Design review of the part built by this model. Coordinates are the model's own, in mm. Face numbers are marked on the shaded views. A direction names the side the tool comes from. Coordinates: 2 decimals unless noted, no trailing zeros. Write each loop counter-clockwise with the first axis right and the second up, starting at its lowest first coordinate (ties: lowest second). Pieces come first, ordered by that corner, then holes.
Q1. For pin 1 Ø2 at (y, z) = (-8.5, -12) entering from -X; pin 2 Ø1 at (x, z) = (-1.5, 6.5) entering from -Y; pin 3 Ø1 at (y, z) = (5, 30) entering from +X, all flat-tipped, find the tip position at first contact; note any pin that passes through.
Q2. Take a section at D-D, the plane x = 6. Write out the cut boundary in (y, z), plus the area to 3 significant figures.
Q3. Take a section at C-C, the plane y = 2.5. Write out the cut boundary in (x, z), plus the area to 3 significant figures.
Q4. For L1, parallel to Y at x = -1.5, z = 33; L2, parallel to Z at x = -4.75, y = 9; L3, parallel to Y at x = -1.9, z = 30.5, list the stretches that pass through material, from the lowest coordinate up.
Q5. For the marked faces 1, 2 and 3, list the 3-axis set-ups (+Z, -Z, +X, -X, +Y, -Y) from which the entire face can be reached by the end or side of a thin tool; tool diameter is ignored.
Q6. Take a section at A-A, the plane z = 61.5. Write out the cut boundary in (x, y).
Q7. Take a section at B-B, the plane z = -12. Write out the cut boundary in (x, y).
from build123d import *

# Parameters (mm, degrees)
SKETCH2_W                                    = 26
SKETCH2_H                                    = 43.2
BOSS_EXTRUDE1_DEPTH                          = 10.1
SKETCH3_R                                    = 1.75
BOSS_EXTRUDE2_DEPTH                          = 7
BOSS_EXTRUDE3_DEPTH                          = 26
BOSS_EXTRUDE4_DEPTH                          = 7
CHAMFER1_SIZE                                = 4.24
CBORE_FOR_M5_HEX_HEAD_CAP_SCREW1_D           = 3.9
CBORE_FOR_M5_HEX_HEAD_CAP_SCREW1_CBORE_D     = 6
CBORE_FOR_M5_HEX_HEAD_CAP_SCREW1_CBORE_DEPTH = 4


with BuildPart() as part:
    # Sketch2 → Boss-Extrude1 (new body)
    with BuildSketch(Plane(origin=(0, 0, 0), x_dir=(0, 0, -1), z_dir=(1, 0, 0))):
        Rectangle(SKETCH2_W, SKETCH2_H)
    extrude(amount=BOSS_EXTRUDE1_DEPTH)

    # Sketch3 → Boss-Extrude2 (add)
    with BuildSketch(Plane.ZY):
        Polygon((-17.5, 15), (17.5, 15), (62.5, 15), (62.5, -15), (17.5, -15), (-17.5, -15), align=None)
        with Locations(Location((12, 9, 0), (0, 0, 304.849904579))):
            Circle(SKETCH3_R, mode=Mode.SUBTRACT)
        with Locations(Location((12, -9, 0), (0, 0, 55.150095421))):
            Circle(SKETCH3_R, mode=Mode.SUBTRACT)
        with Locations(Location((-12, -9, 0), (0, 0, 124.849904579))):
            Circle(SKETCH3_R, mode=Mode.SUBTRACT)
        with Locations(Location((-12, 9, 0), (0, 0, 124.849904579))):
            Circle(SKETCH3_R, mode=Mode.SUBTRACT)
        with Locations(Location((57, -9, 0), (0, 0, 180))):
            Circle(SKETCH3_R, mode=Mode.SUBTRACT)
        with Locations(Location((57, 9, 0), (0, 0, 180))):
            Circle(SKETCH3_R, mode=Mode.SUBTRACT)
        with Locations(Location((33, -9, 0), (0, 0, 180))):
            Circle(SKETCH3_R, mode=Mode.SUBTRACT)
        with Locations(Location((33, 9, 0), (0, 0, 180))):
            Circle(SKETCH3_R, mode=Mode.SUBTRACT)
    extrude(amount=BOSS_EXTRUDE2_DEPTH)

    # Sketch5 → Boss-Extrude3 (add)
    with BuildSketch(Plane(origin=(0, 0, -13), x_dir=(-1, 0, 0), z_dir=(0, 0, -1))):
        Polygon((0, -21.6), (0, -15), (7, -15), align=None)
        Polygon((7, 15), (0, 15), (0, 21.6), align=None)
    extrude(amount=-BOSS_EXTRUDE3_DEPTH)

    # Sketch7 → Boss-Extrude4 (add)
    with BuildSketch(Plane.ZY.offset(7)):
        Polygon((67, -21), (67, 21), (25, 21), (25, 15), (62.5, 15), (62.5, -15), (25, -15), (25, -21), align=None)
    extrude(amount=-BOSS_EXTRUDE4_DEPTH)

    # Chamfer1
    chamfer1_edges = [part.edges().sort_by_distance(p)[0] for p in [
        (-3.5, -21, 25),
        (-3.5, -21, 67),
        (-3.5, 21, 67),
        (-3.5, 21, 25),
    ]]
    chamfer(chamfer1_edges, length=CHAMFER1_SIZE)

    # CBORE for M5 Hex Head Cap Screw1 (through all)
    with Locations(Plane.ZY.offset(7)):
        with Locations((61.5, 15.5), (61.5, -15.5), (30.5, -15.5), (30.5, 15.5)):
            CounterBoreHole(CBORE_FOR_M5_HEX_HEAD_CAP_SCREW1_D / 2, CBORE_FOR_M5_HEX_HEAD_CAP_SCREW1_CBORE_D / 2, CBORE_FOR_M5_HEX_HEAD_CAP_SCREW1_CBORE_DEPTH)


solid = part.part
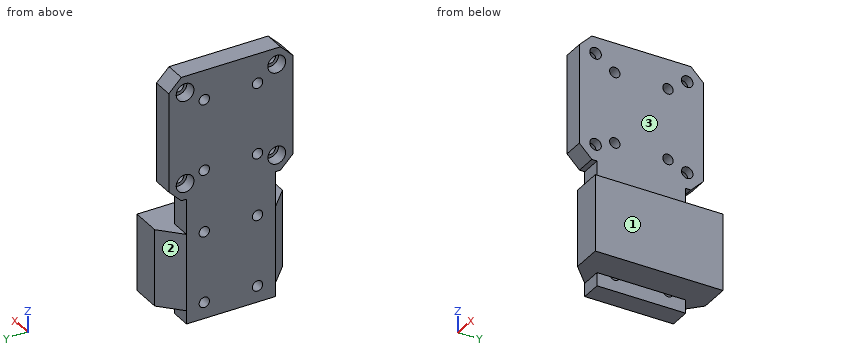
Responses:
1. pin 1: stops at x = 0
1. pin 2: stops at y = -20.66
1. pin 3: stops at x = 0
2. outline: (-21.6, -13) - (21.6, -13) - (21.6, 13) - (-21.6, 13) - close
2. area: 1,120 mm2
3. outline: (-7, -17.5) - (0, -17.5) - (0, -13) - (10.1, -13) - (10.1, 13) - (0, 13) - (0, 67) - (-7, 67) - close
3. area: 854 mm2
4. L1: y = -21 to -10.75, -7.25 to 7.25, 10.75 to 21
4. L2: z = -17.5 to -13.75, -10.25 to 10.25, 13.75 to 31.25, 34.75 to 55.25, 58.75 to 67
4. L3: y = -21 to -17.45, -13.55 to 13.55, 17.45 to 21
5. face 1: +Z, -Z, +X, +Y, -Y
5. face 2: -Z, -X, +Y
5. face 3: +Z, +X, +Y, -Y
6. outline: (-7, -21) - (0, -21) - (0, -17.45) - (-3, -17.45) - (-3, -18.5) - (-7, -18.5) - close; (-7, -12.5) - (-3, -12.5) - (-3, -13.55) - (0, -13.55) - (0, 13.55) - (-3, 13.55) - (-3, 12.5) - (-7, 12.5) - close; (-7, 18.5) - (-3, 18.5) - (-3, 17.45) - (0, 17.45) - (0, 21) - (-7, 21) - close
7. outline: (-7, -15) - (0, -21.6) - (10.1, -21.6) - (10.1, 21.6) - (0, 21.6) - (-7, 15) - (-7, 10.75) - (0, 10.75) - (0, 7.25) - (-7, 7.25) - (-7, -7.25) - (0, -7.25) - (0, -10.75) - (-7, -10.75) - close
